For this review, use the dimensioned drawing (mm, ordinates from the lowest corner) and the shaded views. A direction names the side the tool comes from. Coordinates: 2 decimals unless noted, no trailing zeros. Write each loop counter-clockwise with the first axis right and the second up, starting at its lowest first coordinate (ties: lowest second). Pieces come first, ordered by that corner, then holes.
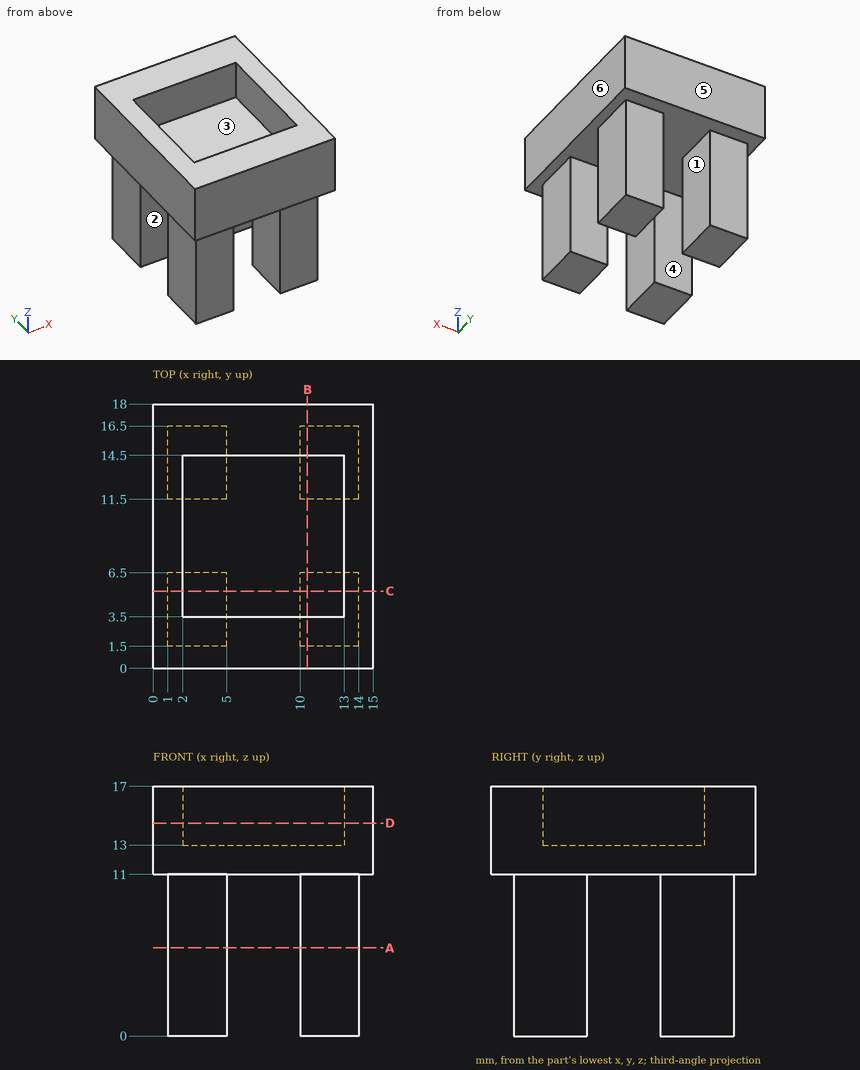
(1) Consider section D-D (z = 14.5). Give the boundary of the cut face in (x, y), plus the area to 3 significant figures.
(2) Mouldability with a two-part tool opening along Y and no side actions: class the marked faces 4, 5 and 6 as +Y half, -Y half, draft (parallel to the pull), parting line (faces both ways), or undercut.
(3) Insertion check: pin 1 Ø3 at (x, z) = (3.5, 3) entering from -Y; pin 2 Ø5.5 at (y, z) = (14, 7) entering from +X; pin 3 Ø3 at (x, z) = (11.5, 3) entering from +Y; pin 4 Ø1 at (y, z) = (8, 4) entering from +X. Each pin has a flat end and moves straight along its axis. Give the tip position at first contact, or say it passes through.
(4) Wall thickness on line 1 (Y direction, x = 13.75, z = 6.75); line 2 (X direction, y = 2, z = 1.5); line 3 (Z direction, x = 10, y = 11): over which ranges is each line inside the solid? List them lowest first.
(5) Consider section B-B (x = 10.5). Give the boundary of the cut face in (y, z).
(6) For the marked faces 1, 2 and 3, list the 3-axis set-ups (+Z, -Z, +X, -X, +Y, -Y) from which the entire face can be reached by the end or side of a thin tool; tool diameter is ignored.
(7) Consider section C-C (y = 5.25). Give the boundary of the cut face in (x, z).
(8) Consider section A-A (z = 6). Give the boundary of the cut face in (x, y), plus the area to 3 significant figures.
Results:
1. outline: (0, 0) - (15, 0) - (15, 18) - (0, 18) - close; hole (2, 3.5) - (13, 3.5) - (13, 14.5) - (2, 14.5) - close
1. area: 149 mm2
2. face 4: undercut
2. face 5: +Y half
2. face 6: draft
3. pin 1: stops at y = 1.5
3. pin 2: stops at x = 14
3. pin 3: stops at y = 16.5
3. pin 4: passes through
4. line 1: y = 1.5 to 6.5, 11.5 to 16.5
4. line 2: x = 1 to 5, 10 to 14
4. line 3: z = 11 to 13
5. outline: (0, 11) - (1.5, 11) - (1.5, 0) - (6.5, 0) - (6.5, 11) - (11.5, 11) - (11.5, 0) - (16.5, 0) - (16.5, 11) - (18, 11) - (18, 17) - (14.5, 17) - (14.5, 13) - (3.5, 13) - (3.5, 17) - (0, 17) - close
6. face 1: -Z, +Y, -Y
6. face 2: -Z, +X, -X
6. face 3: +Z
7. outline: (0, 11) - (1, 11) - (1, 0) - (5, 0) - (5, 11) - (10, 11) - (10, 0) - (14, 0) - (14, 11) - (15, 11) - (15, 17) - (13, 17) - (13, 13) - (2, 13) - (2, 17) - (0, 17) - close
8. outline: (1, 1.5) - (5, 1.5) - (5, 6.5) - (1, 6.5) - close; (1, 11.5) - (5, 11.5) - (5, 16.5) - (1, 16.5) - close; (10, 1.5) - (14, 1.5) - (14, 6.5) - (10, 6.5) - close; (10, 11.5) - (14, 11.5) - (14, 16.5) - (10, 16.5) - close
8. area: 80.0 mm2
